```python
from build123d import *

# Parameters (mm, degrees)
SKETCH1_R           = 2.85
BOSS_EXTRUDE1_DEPTH = 3
SKETCH2_R           = 1.5
BOSS_EXTRUDE2_DEPTH = 20
CHAMFER1_SIZE       = 0.3
CUT_EXTRUDE1_DEPTH  = 2


with BuildPart() as part:
    # Sketch1 → Boss-Extrude1 (new body)
    with BuildSketch(Plane.XY):
        Circle(SKETCH1_R)
    extrude(amount=BOSS_EXTRUDE1_DEPTH)

    # Sketch2 → Boss-Extrude2 (add)
    with BuildSketch(Plane(origin=(0, 0, 0), x_dir=(-1, 0, 0), z_dir=(0, 0, -1))):
        Circle(SKETCH2_R)
    extrude(amount=BOSS_EXTRUDE2_DEPTH)

    # Chamfer1
    chamfer1_edges = [part.edges().sort_by_distance(p)[0] for p in [
        (1.5, 0, -20),
    ]]
    chamfer(chamfer1_edges, length=CHAMFER1_SIZE)

    # Sketch3 → Cut-Extrude1 (cut)
    with BuildSketch(Plane.XY.offset(3)):
        Polygon((0, 1.443375673), (-1.25, 0.721687836), (-1.25, -0.721687836), (0, -1.443375673), (1.25, -0.721687836), (1.25, 0.721687836), align=None)
    extrude(amount=-CUT_EXTRUDE1_DEPTH, mode=Mode.SUBTRACT)


solid = part.part
```
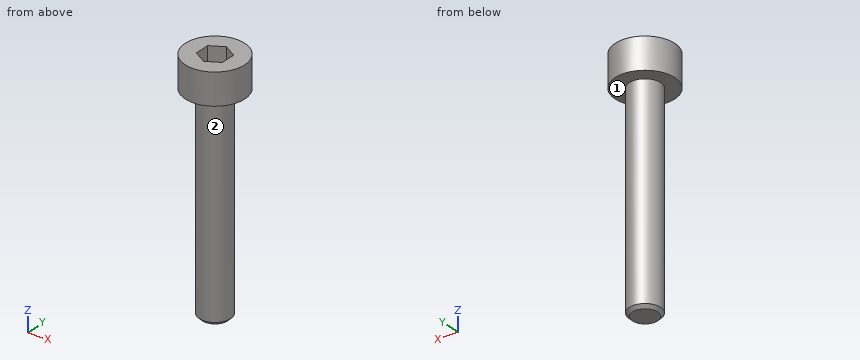
Verification items for the finished model (mm, model axes). Face numbers are marked on the shaded views. Coordinates: 2 decimals unless noted, no trailing zeros. Loops run counter-clockwise (first coordinate to the right, second up) from the corner with the lowest first, then second, coordinate; pieces in that order, holes last. Notation, with made-up numbers: (10, 53.5) -> (52, 53.5) arc R23 ccw to (52, 68.5) -> close; hole circle Ø2 at (-28.5, -30). An arc over 180 degrees is marked (long way). Answer in a Markdown table with one row per item.
1) Scan lines: line 1 along Z through (x, y) = (1.2, -1.7); line 2 along Z through (x, y) = (-0.1, 0.45); line 3 along X through (y, z) = (-1, -2.5). Record each from-to range of solid material in increasing order. Write a range as from..to.
The answers:
| item | result |
|---|---|
| line 1 | z = 0..3 |
| line 2 | z = -20..1 |
| line 3 | x = -1.12..1.12 |
2) Section check A-A (y = 0). Record the cut outline in (x, z), and give its area (3 significant figures).
The answers:
| item | result |
|---|---|
| outline | (-2.85, 0) -> (-1.5, 0) -> (-1.5, -19.7) -> (-1.2, -20) -> (1.2, -20) -> (1.5, -19.7) -> (1.5, 0) -> (2.85, 0) -> (2.85, 3) -> (1.25, 3) -> (1.25, 1) -> (-1.25, 1) -> (-1.25, 3) -> (-2.85, 3) -> close |
| area | 72.0 mm2 |
3) Section check B-B (z = -14.25). Record the cut outline in (x, y), and give its area (3 significant figures).
The answers:
| item | result |
|---|---|
| outline | circle Ø3 at (0, 0) |
| area | 7.07 mm2 |
4) Draft check along Y on the marked faces 1 and 2. Enter one of: released by +Y, released by -Y, zero draft, split by the parting line, or undercut.
The answers:
| item | result |
|---|---|
| face 1 | zero draft |
| face 2 | split by the parting line |
5) Section check C-C (y = 2.25). Record the cut outline in (x, z).
The answers:
| item | result |
|---|---|
| outline | (-1.75, 0) -> (1.75, 0) -> (1.75, 3) -> (-1.75, 3) -> close |
6) Depth check by flat-ended pin: P1, Ø1.5, axis at x = -1.5, z = -2.5, coming from the +Y side; P2, Ø2, axis at x = 0, y = -0.5, coming from the +Z side; P3, Ø3, axis at x = 1, z = -12, coming from the +Y side; P4, Ø1, axis at x = -1.5, y = -1.5, coming from the -Z side. Enter the tip coordinate at first touch or a pass-through.
The answers:
| item | result |
|---|---|
| P1 | stops at y = 1.3 |
| P2 | stops at z = 3 |
| P3 | stops at y = 1.5 |
| P4 | stops at z = 0 |
